Read the model definition and answer for the solid it produces. Units are mm, in the model's axes. A direction names the side the tool comes from. Coordinates: 2 decimals unless noted, no trailing zeros. Write each loop counter-clockwise with the first axis right and the second up, starting at its lowest first coordinate (ties: lowest second). Pieces come first, ordered by that corner, then holes. Notation, with made-up numbers: (87, 1) - (143, 1) arc R21 ccw to (143, 33) - close; hole circle Ø7 at (0.5, -30.5). An arc over 180 degrees is marked (long way). Return JSON: item names as keys, results as strings.
```python
from build123d import *


with BuildPart() as part:
    # AdditivePipe: sweep along a path in Sketch
    with BuildLine(Plane.XY) as additivepipe_path:
        Line((0, 0), (0, 50))
        ThreePointArc((0, 50), (-63.5, 113.5), (-127, 50))
        Line((-127, 50), (-127, 40))
    # Sketch001 → AdditivePipe (sweep)
    with BuildSketch(Plane.XZ):
        Polygon((2.1, 0), (0.449013, 0.449013), (0, 2.1), (-0.449013, 0.449013), (-2.1, 0), (-0.449013, -0.449013), (0, -2.1), (0.449013, -0.449013), align=None)
    sweep(path=additivepipe_path.line)


solid = part.part
```
(1) A cutting plane is placed at B-B (y = 12). Determine the outline of the cut face in (x, z), and give its area (3 significant figures).
Answer:
{"outline": "(-2.1, 0) - (-0.45, -0.45) - (0, -2.1) - (0.45, -0.45) - (2.1, 0) - (0.45, 0.45) - (0, 2.1) - (-0.45, 0.45) - close", "area": "3.77 mm²"}
(2) Which of the six approach directions +Z, -Z, +X, -X, +Y, -Y give full straight-line access (tool end or side, diameter ignored) to faces 1 (the face through (-127, 40, 0)), 2 (the face through (0, 0, 0))?
Answer:
{"face 1": "+Z, -Z, -X, -Y", "face 2": "+Z, -Z, +X, -X, -Y"}
(3) Straight lines are drawn through the part: line 1 (X direction, y = 47, z = -1.25); line 2 (X direction, y = 97.5, z = 1.7); line 3 (Y direction, x = -119, z = -0.75). For each, find the intervals that lie inside material, in ascending order. Write a range as from..to.
Answer:
{"line 1": "-127.23..-126.77, -0.23..0.23", "line 2": "-105.81..-105.48, -21.52..-21.19", "line 3": "80.09..81.6"}
(4) Flat-ended cylindrical pins translate along their axes: P1, Ø10, axis at x = -18.5, y = 80.5, coming from the -Z side (1 decimal); P2, Ø1.3, axis at x = -127, z = 0.5, coming from the -Y side; P3, Ø1, axis at x = -57.5, z = 1.5, coming from the +Y side. Find the tip coordinate at first contact, or state that the pin passes through.
Answer:
{"P1": "through", "P2": "y = 40", "P3": "y = 113.52"}
(5) A cutting plane is placed at A-A (x = -63.5). Determine the outline of the cut face in (y, z).
Answer:
{"outline": "(111.4, 0) - (113.05, -0.45) - (113.5, -2.1) - (113.95, -0.45) - (115.6, 0) - (113.95, 0.45) - (113.5, 2.1) - (113.05, 0.45) - close"}
